Here's the drawing with two shaded views (mm, measured from the low corner). I have some questions. A direction names the side the tool comes from. Give positions to 0.01 mm unless a question says otherwise; leave off trailing zeros. Loops run counter-clockwise (first coordinate to the right, second up) from the corner with the lowest first, then second, coordinate; pieces in that order, holes last. Notation, with made-up numbers: M -21,-16.75 L 30,-16.75 A7 ccw 30,-8.75 Z; hole C 61,77 d2. An arc over 180 degrees is marked long. Answer in a Markdown table with one row per item. Add a question column.
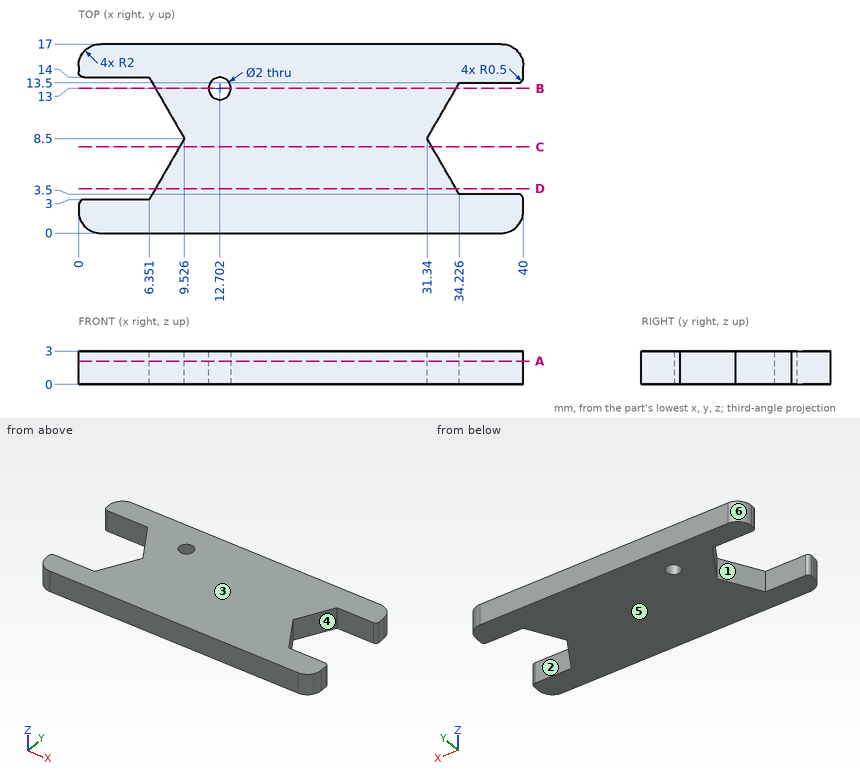
Item 1: Suppose I cut it at B-B (y = 13). List the corners of the cut face in (x, z) for me.
Item 2: For P1, Ø1.5, axis at y = 4.5, z = 1, coming from the +X side, with a flat end and sliding along its axis, tell me the tip position at first contact or that it passes through.
Item 3: I need wall thicknesses on L1, parallel to Y at x = 5, z = 1.85; L2, parallel to Y at x = 8, z = 1.1 (1 decimal); L3, parallel to X at y = 7.75, z = 2.7 (1 decimal). Which ranges of each line are inside material? Lowest first, please.
Item 4: Suppose I cut it at D-D (y = 4). List the corners of the cut face in (x, z) for me.
Item 5: For the marked faces 1, 2 and 3, which set-ups out of +Z, -Z, +X, -X, +Y, -Y let a thin tool reach every point of the face, with its end or its side?
Item 6: If we mould it in two halves opening along Y, with no side actions, what happens to the marked faces 4, 5 and 6? For each: +Y half, -Y half, draft (parallel to the pull), parting line (faces both ways), or undercut.
Item 7: Suppose I cut it at C-C (y = 7.75). List the corners of the cut face in (x, z) for me.
Item 8: Suppose I cut it at A-A (z = 2.1). List the corners of the cut face in (x, y) for me, then the cut area to 3 significant figures.
Values found:
| question | item | result |
|---|---|---|
| 1 | outline | M 6.93,0 L 11.7,0 L 11.7,3 L 6.93,3 Z; M 13.7,0 L 33.94,0 L 33.94,3 L 13.7,3 Z |
| 2 | P1 | x = 34.08 |
| 3 | L1 | 0 to 3, 14 to 17 |
| 3 | L2 | 0 to 5.9, 11.1 to 17 |
| 3 | L3 | 9.1 to 31.8 |
| 4 | outline | M 6.93,0 L 33.94,0 L 33.94,3 L 6.93,3 Z |
| 5 | face 1 | +Z, -Z, -X |
| 5 | face 2 | +Z, -Z, +X |
| 5 | face 3 | +Z, +X, -X, +Y, -Y |
| 6 | face 4 | undercut |
| 6 | face 5 | draft |
| 6 | face 6 | +Y half |
| 7 | outline | M 9.09,0 L 31.77,0 L 31.77,3 L 9.09,3 Z |
| 8 | outline | M 0,2 A2 ccw 2,0 L 38,0 A2 ccw 40,2 L 40,3 A0.5 ccw 39.5,3.5 L 34.23,3.5 L 31.34,8.5 L 34.23,13.5 L 39.5,13.5 A0.5 ccw 40,14 L 40,15 A2 ccw 38,17 L 2,17 A2 ccw 0,15 L 0,14.5 A0.5 ccw 0.5,14 L 6.35,14 L 9.53,8.5 L 6.35,3 L 0.5,3 A0.5 ccw 0,2.5 Z; hole C 12.7,13 d2 |
| 8 | area | 514 mm² |
